from build123d import *

# Parameters (mm, degrees)
F0_W        = 100
F0_H        = 100
F1_DEPTH    = 20
F2_W        = 100
F2_H        = 20
F3_DEPTH    = 80
F4_R        = 15
F5_DEPTH    = 20
F6_T1_DEPTH = 195
F7_W        = 30
F7_H        = 80
F8_DEPTH    = 80
F9_SIZE     = 80
F10_W       = 40
F10_H       = 40
F11_DEPTH   = 20


# Not quite as in the source:
# - a fillet or chamfer that OpenCascade refuses, or shapes differently, is made with other operations: its cross-section is extruded or revolved along the edge and cut away or added


with BuildPart() as f1:
    # F0 (on Top) → F1 (new body)
    with BuildSketch(Plane.XY):
        Rectangle(F0_W, F0_H)
    extrude(amount=F1_DEPTH)

    # F2 (on face) → F3 (join)
    with BuildSketch(Plane.XY.offset(20)):
        with Locations((0, 40)):
            Rectangle(F2_W, F2_H)
    extrude(amount=F3_DEPTH)

    # F4 (on face) → F5 (cut)
    with BuildSketch(Plane.XY.offset(20)):
        with Locations((-25, -25)):
            Circle(F4_R)
    extrude(amount=-F5_DEPTH, mode=Mode.SUBTRACT)

    # F6: fillet of radius 35 on 1 edges, made by hand

    # F6_s2 → F6_t1 (cut)
    with BuildSketch(Plane.XY.offset(-87.5)):
        with BuildLine():
            add(Edge.make_bspline(
                [(-50, -15), (-50, -50), (-15, -50)],
                knots=[0, 0, 0, 1, 1, 1], degree=2, weights=[1, 1, 1]))
            Line((-15, -50), (-50, -50))
            Line((-50, -50), (-50, -15))
        make_face()
    extrude(amount=F6_T1_DEPTH, mode=Mode.SUBTRACT)

    # F7 (on face) → F8 (join)
    with BuildSketch(Plane.XY.offset(20)):
        with Locations((35, -10)):
            Rectangle(F7_W, F7_H)
    extrude(amount=F8_DEPTH)

    # F9
    f9_edges = [f1.edges().sort_by_distance(p)[0] for p in [
        (35, -50, 100),
    ]]
    chamfer(f9_edges, length=F9_SIZE)

    # F10 (on face) → F11 (cut)
    with BuildSketch(Plane.XZ.offset(-30)):
        with Locations((-15, 60)):
            Rectangle(F10_W, F10_H)
    extrude(amount=-F11_DEPTH, mode=Mode.SUBTRACT)


solid = f1.part
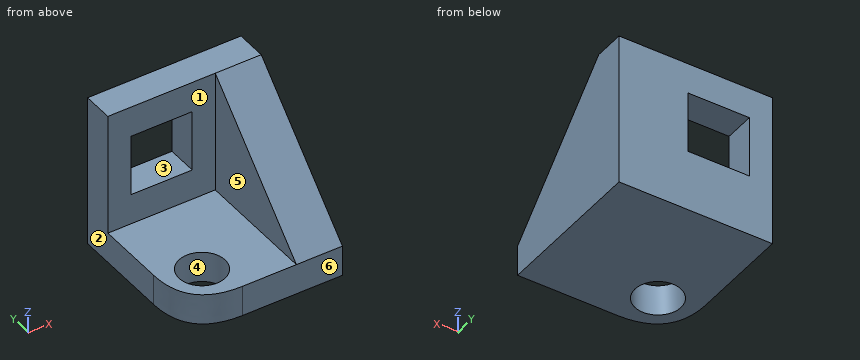
Part model, mm, in its own coordinate system. Face numbers are marked on the shaded views. A direction names the side the tool comes from. Round coordinates to 2 decimals unless told otherwise and drop trailing zeros. Write each loop counter-clockwise with the first axis right and the second up, starting at its lowest first coordinate (ties: lowest second). Pieces come first, ordered by that corner, then holes. Notation, with made-up numbers: (62, -12) - (97, -12) arc R22 ccw to (97, 16) - close; hole circle Ø8 at (31, 12.25). An arc over 180 degrees is marked (long way). Use CSV: the item, a comma, the result in double quotes.
Item 1: Slice it at C-C, the plane x = 44. Write the cut outline in (y, z), then the cut area to 3 significant figures.
Results list:
outline,"(-50, 0) - (50, 0) - (50, 100) - (30, 100) - (-50, 20) - close"
area,"6,800 mm²"
Item 2: Tool access for the marked faces 1, 2 and 3: list every direction of +Z, -Z, +X, -X, +Y, -Y with a clear straight run to the whole face (end or side of a thin tool).
Results list:
face 1,"+Z, -X, -Y"
face 2,"+Z, -Z, -X, +Y, -Y"
face 3,"+Y, -Y"
Item 3: Pull direction X, two halves, no side cores. Call the marked faces 4, 5 and 6: pulls with the +X half, pulls with the -X half, needs draft (parallel to the pull), parting line crosses it, or undercut.
Results list:
face 4,"undercut"
face 5,"pulls with the -X half"
face 6,"needs draft"
Item 4: Wall check: L1, parallel to Z at x = -1, y = 25.5; L2, parallel to Z at x = -4, y = 44; L3, parallel to Y at x = -25, z = 10. Give the ranges that are in metal, low to high.
Results list:
L1,"z = 0 to 20"
L2,"z = 0 to 40, 80 to 100"
L3,"y = -49.16 to -40, -10 to 50"
Item 5: Slice it at A-A, the plane z = 68.5. Write the cut outline in (x, y).
Results list:
outline,"(-50, 30) - (-35, 30) - (-35, 50) - (-50, 50) - close; (5, 30) - (20, 30) - (20, -1.5) - (50, -1.5) - (50, 50) - (5, 50) - close"
Item 6: Flat gauge pins, fed straight in: P1, Ø3, axis at x = -10, z = 40.5, coming from the +Y side; P2, Ø6, axis at x = -24, z = 90, coming from the -Y side; P3, Ø4, axis at y = -23, z = 32, coming from the -X side; P4, Ø21, axis at x = -25.5, y = -3, coming from the +Z side. Where does each tip first touch, or does it go through?
Results list:
P1,"stops at y = 50"
P2,"stops at y = 30"
P3,"stops at x = 20"
P4,"stops at z = 20"
Item 7: Slice it at B-B, the plane y = 33. Write the cut outline in (x, z).
Results list:
outline,"(-50, 0) - (50, 0) - (50, 100) - (-50, 100) - close; hole (-35, 40) - (5, 40) - (5, 80) - (-35, 80) - close"
Item 8: Slice it at D-D, the plane y = 22.5. Write the cut outline in (x, z).
Results list:
outline,"(-50, 0) - (50, 0) - (50, 92.5) - (20, 92.5) - (20, 20) - (-50, 20) - close"
